Work out the finished part from the listing and answer in its coordinate system (mm). Face numbers are marked on the shaded views. A direction names the side the tool comes from. Round coordinates to 2 decimals unless told otherwise and drop trailing zeros. Write each loop counter-clockwise with the first axis right and the second up, starting at its lowest first coordinate (ties: lowest second). Pieces come first, ordered by that corner, then holes. Notation, with made-up numbers: M -7,42 L 43,42 A15 cw 43,49 Z; hole C -39,37 d6. An arc over 180 degrees is marked long. Answer in a Markdown table with one row per item.
```python
from build123d import *

# Parameters (mm, degrees)
SKETCH_1_W          = 4
SKETCH_1_H          = 3.5
SKETCH_2_R          = 2
EXTRUDE_1_DEPTH     = 16
CUT_EXTRUDE_1_DEPTH = 2
CHAMFER_1_SIZE      = 0.6062
CHAMFER_1_SIZE2     = 0.35
FILLET_1_R          = 0.2


with BuildPart() as part:
    # 草图1 → 旋转1 (revolve)
    with BuildSketch(Plane.XY):
        with Locations((2, 1.75)):
            Rectangle(SKETCH_1_W, SKETCH_1_H)
    revolve(axis=Axis((0, 0, 0), (1, 0, 0)))

    # 草图2 → 凸台-拉伸1 (add)
    with BuildSketch(Plane(origin=(4, 0, 0), x_dir=(0, 0, -1), z_dir=(1, 0, 0))):
        Circle(SKETCH_2_R)
    extrude(amount=EXTRUDE_1_DEPTH)

    # 草图3 → 切除-拉伸1 (cut)
    with BuildSketch(Plane.ZY):
        Polygon((0, 1.72), (-1.489563695, 0.86), (-1.489563695, -0.86), (0, -1.72), (1.489563695, -0.86), (1.489563695, 0.86), align=None)
    extrude(amount=-CUT_EXTRUDE_1_DEPTH, mode=Mode.SUBTRACT)

    # 倒角1
    chamfer_1_edges = [part.edges().sort_by_distance(p)[0] for p in [
        (20, 0, 2),
    ]]
    chamfer_1_side = [part.faces().sort_by_distance(p)[0] for p in [
        (20, 0, 0),
    ]]
    chamfer(chamfer_1_edges, length=CHAMFER_1_SIZE, length2=CHAMFER_1_SIZE2, reference=chamfer_1_side[0])

    # 圆角1
    fillet_1_edges = [part.edges().sort_by_distance(p)[0] for p in [
        (0, -3.5, 0),
        (4, 0, 2),
    ]]
    fillet(fillet_1_edges, radius=FILLET_1_R)


solid = part.part
```
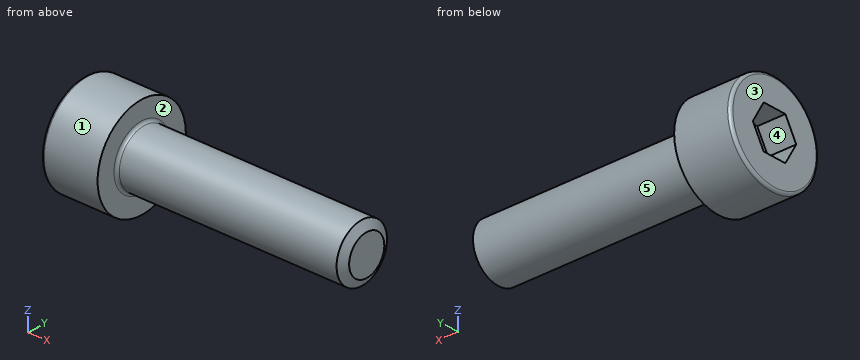
1. A tool of negligible diameter and unlimited length cuts with its end or side. For the marked faces 1 and 2, from which of +Z, -Z, +X, -X, +Y, -Y can it reach the whole face along a straight path? Write none if from no direction.
Calculated:
| item | result |
|---|---|
| face 1 | +X, -X |
| face 2 | +X |
2. Determine the mould class of the marked faces 3, 4 and 5 for opening direction Y: released by +Y, released by -Y, zero draft, split by the parting line, or undercut.
Calculated:
| item | result |
|---|---|
| face 3 | zero draft |
| face 4 | undercut |
| face 5 | split by the parting line |
3. Consider line 1 along X through (y, z) = (-2.5, 2); line 2 along Z through (x, y) = (17.75, -1.75); line 3 along Z through (x, y) = (3.5, 0.25). Determine where each line is inside the solid, lowest interval first. Write a range as from..to.
Calculated:
| item | result |
|---|---|
| line 1 | x = 0..4 |
| line 2 | z = -0.97..0.97 |
| line 3 | z = -3.49..3.49 |
4. The part is cut by section C-C (x = 10.5). Determine the outline of the cut face in (y, z), plus the area to 3 significant figures.
Calculated:
| item | result |
|---|---|
| outline | C 0,0 d4 |
| area | 12.6 mm² |
5. The part is cut by section B-B (y = 0). Determine the outline of the cut face in (x, z).
Calculated:
| item | result |
|---|---|
| outline | M 0,-3.3 A0.2 ccw 0.2,-3.5 L 4,-3.5 L 4,-2.2 A0.2 cw 4.2,-2 L 19.65,-2 L 20,-1.39 L 20,1.39 L 19.65,2 L 4.2,2 A0.2 cw 4,2.2 L 4,3.5 L 0.2,3.5 A0.2 ccw 0,3.3 L 0,1.49 L 2,1.49 L 2,-1.49 L 0,-1.49 Z |
6. Given pin 1 (1 mm diameter, centred on x = 10, z = -2, fed in from +Y); pin 2 (2 mm diameter, centred on x = 11, z = -0.5, fed in from +Y); pin 3 (1 mm diameter, centred on x = 12.5, y = -2, fed in from +Z), each flat-ended and moving along its own axis, determine where each tip first touches the part or whether it passes through.
Calculated:
| item | result |
|---|---|
| pin 1 | stops at y = 1.32 |
| pin 2 | stops at y = 2 |
| pin 3 | stops at z = 1.32 |
7. The part is cut by section A-A (x = 1.75). Determine the outline of the cut face in (y, z).
Calculated:
| item | result |
|---|---|
| outline | C 0,0 d7; hole M -1.72,0 L -0.86,-1.49 L 0.86,-1.49 L 1.72,0 L 0.86,1.49 L -0.86,1.49 Z |
